Read the model definition and answer for the solid it produces. Units are mm, in the model's axes. Coordinates: 2 decimals unless noted, no trailing zeros. Write each loop counter-clockwise with the first axis right and the second up, starting at its lowest first coordinate (ties: lowest second). Pieces come first, ordered by that corner, then holes. Notation, with made-up numbers: (25, -39.5) -> (63, -39.5) arc R20 cw to (63, -8.5) -> close; hole circle Ø9 at (21.25, 85). An arc over 180 degrees is marked (long way). Write item = value, one per line. Start each with the question number.
1) Section A-A (z = 29) is taken. Determine the outline of the cut face in (x, y).
2) Find the intervals of material crossed by line 1 along X through (y, z) = (20.5, 15); line 2 along Z through (x, y) = (62, -83); line 3 along X through (y, z) = (-37, 37.5), in increasing order. Write a range as from..to.
3) Section C-C (y = 72) is taken. Determine the outline of the cut face in (x, z).
4) Flat-ended cylindrical pins translate along their axes: pin 1 Ø5 at (x, y) = (22.5, -88.5) entering from -Z; pin 2 Ø2 at (x, z) = (-15, 140.5) entering from +Y; pin 3 Ø4 at (y, z) = (6.5, 143) entering from -X; pin 4 Ø3 at (x, z) = (-69.5, 167) entering from -Y. Find the tip coordinate at first contact, or state that the pin passes through.
5) Section B-B (x = 46.5) is taken. Determine the outline of the cut face in (y, z).
6) Section D-D (x = -20) is taken. Determine the outline of the cut face in (y, z), plus the area to 3 significant figures.
from build123d import *

# Parameters (mm, degrees)
SKETCH1_R           = 152.4
BOSS_EXTRUDE1_DEPTH = 300
CIRPATTERN1_COUNT   = 3


with BuildPart() as part:
    # Sketch1 → Boss-Extrude1 (new body)
    with BuildSketch(Plane.XY):
        Circle(SKETCH1_R)
    extrude(amount=BOSS_EXTRUDE1_DEPTH)

    # Sketch2 → Cut-Revolve1 (revolve, cut)
    with BuildSketch(Plane(origin=(0, 0, -90.9), x_dir=(-0.64278761, 0.766044443, 0), z_dir=(0.766044443, 0.64278761, 0))):
        with BuildLine():
            Line((-144.337567297, -293.6), (-144.337567297, -593.6))
            ThreePointArc((-144.337567297, -593.6), (465.662432703, 16.4), (-144.337567297, 626.4))
            Line((-144.337567297, 626.4), (-144.337567297, 326.4))
            ThreePointArc((-144.337567297, 326.4), (165.662432703, 16.4), (-144.337567297, -293.6))
        make_face()
    cut_revolve1 = revolve(axis=Axis((92.778399871, -110.568991361, -112.7), (0, 0, 1)), mode=Mode.SUBTRACT)

    # CirPattern1: Cut-Revolve1 ×3 about axis
    cirpattern1_axis = Axis((0, 0, 0), (0, 0, 1))
    for i in range(1, CIRPATTERN1_COUNT):
        add(cut_revolve1.rotate(cirpattern1_axis, i * 360 / CIRPATTERN1_COUNT), mode=Mode.SUBTRACT)


solid = part.part
Answer key:
q1.outline = (-132.04, 76.09) arc R152.4 ccw to (-98.06, -116.67) arc R292.21 ccw to (0.12, -152.4) arc R152.4 ccw to (150.06, -26.59) arc R292.21 ccw to (131.92, 76.31) arc R152.4 ccw to (-52.01, 143.25) arc R292.21 ccw to start
q2.line_1 = -151.01..151.01
q2.line_2 = 0..144.91
q2.line_3 = -147.84..146.67
q3.outline = (-134.32, 0) -> (134.32, 0) -> (134.32, 26.72) arc R294.41 ccw to (26.21, 167.03) arc R250.54 ccw to (-134.32, 31.31) -> close
q4.pin_1 = 0
q4.pin_2 = 86.25
q4.pin_3 = -97.15
q4.pin_4 = -20.74
q5.outline = (-145.13, 0) -> (145.13, 0) -> (145.13, 94.54) arc R306.53 ccw to (127.76, 118.27) arc R245.99 ccw to (-55.42, 169.61) arc R309.99 ccw to (-145.13, 56.89) -> close
q6.outline = (-151.08, 0) -> (151.08, 0) -> (151.08, 47.65) arc R288.76 ccw to (-3.53, 193.68) arc R302.14 ccw to (-151.08, 20.8) -> close
q6.area = 40,800 mm^2
